from build123d import *

# Parameters (mm, degrees)
F0_R          = 13.5
F0_R_2        = 11.95
F1_DEPTH      = 3.6
F1_DEPTH_BACK = 3.992162
F2_R          = 12.1
F2_R_2        = 11.95
F3_DEPTH      = 2.4
F4_R          = 12.1
F5_DEPTH      = 2.4


with BuildPart() as f1:
    # F0 (on Front) → F1 (new body, two sides)
    with BuildSketch(Plane.XZ) as f1_sk:
        Circle(F0_R)
        Circle(F0_R_2, mode=Mode.SUBTRACT)
    extrude(amount=F1_DEPTH)
    extrude(f1_sk.sketch, amount=-F1_DEPTH_BACK)

    # F2 (on face) → F3 (cut)
    with BuildSketch(Plane.XZ.offset(3.6)):
        Circle(F2_R)
        Circle(F2_R_2, mode=Mode.SUBTRACT)
    extrude(amount=-F3_DEPTH, mode=Mode.SUBTRACT)

    # F4 (on face) → F5 (cut)
    with BuildSketch(Plane(origin=(0, 3.992162, 0), x_dir=(-1, 0, 0), z_dir=(0, 1, 0))):
        Circle(F4_R)
    extrude(amount=-F5_DEPTH, mode=Mode.SUBTRACT)


solid = f1.part
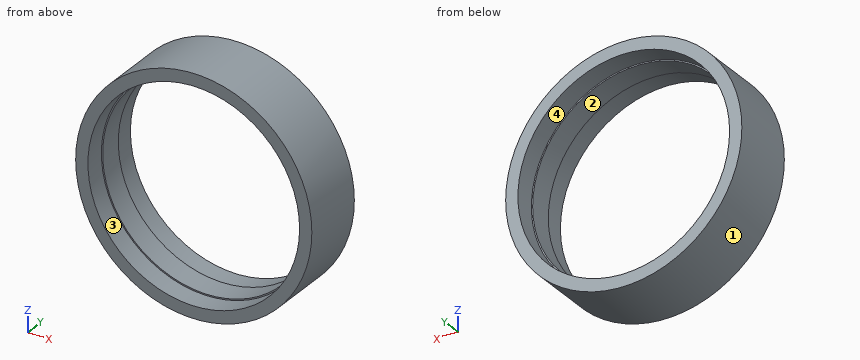
For this review, take the finished solid that the model builds, in its own axes (mm). Face numbers are marked on the shaded views. A direction names the side the tool comes from. Round coordinates to 2 decimals unless told otherwise and drop trailing zeros. Loops run counter-clockwise (first coordinate to the right, second up) from the corner with the lowest first, then second, coordinate; pieces in that order, holes last. Notation, with made-up numbers: (16, 67) - (44, 67) arc R18 ccw to (44, 97) - close; hole circle Ø6 at (3.5, -4.5). An arc over 180 degrees is marked (long way). One line per item, written item: value. Start each with the question number.
Item 1: The part is to be moulded in two halves that separate along X. For the marked faces 1 and 2, say which applies: +X half, -X half, draft (parallel to the pull), parting line (faces both ways), or undercut.
Item 2: For L1, parallel to Z at x = 0, y = 2.1; L2, parallel to Z at x = -9.75, y = -2.5; L3, parallel to X at y = 1.75, z = -1, list the stretches that pass through material, from the lowest coordinate up.
Item 3: Take a section at A-A (z = 0). Give the boundary of the cut face in (x, y).
Item 4: For the marked faces 3 and 4, list the 3-axis set-ups (+Z, -Z, +X, -X, +Y, -Y) from which the entire face can be reached by the end or side of a thin tool; tool diameter is ignored.
Item 5: Take a section at B-B (x = -1). Give the boundary of the cut face in (y, z), plus the area to 3 significant figures.
Item 6: Take a section at C-C (y = 3.25). Give the boundary of the cut face in (x, z).
Item 7: Clearance check with flat-ended pins moving along their axes: pin 1 Ø1.5 at (x, z) = (0, -11) entering from -Y; pin 2 Ø1 at (y, z) = (1.5, -9) entering from +X; pin 3 Ø1.5 at (x, y) = (7, -2) entering from +Z. State where each tip first meets the part, or that it passes through.
Item 8: Take a section at D-D (y = 0.5). Give the boundary of the cut face in (x, z).
Answer below:
1. face 1: parting line
1. face 2: undercut
2. L1: z = -13.5 to -12.1, 12.1 to 13.5
2. L2: z = -9.34 to -7.17, 7.17 to 9.34
2. L3: x = -13.46 to -12.06, 12.06 to 13.46
3. outline: (-13.5, -3.6) - (-12.1, -3.6) - (-12.1, -1.2) - (-11.95, -1.2) - (-11.95, 1.59) - (-12.1, 1.59) - (-12.1, 3.99) - (-13.5, 3.99) - close; (11.95, -1.2) - (12.1, -1.2) - (12.1, -3.6) - (13.5, -3.6) - (13.5, 3.99) - (12.1, 3.99) - (12.1, 1.59) - (11.95, 1.59) - close
4. face 3: -Y
4. face 4: +Y
5. outline: (-3.6, -13.46) - (3.99, -13.46) - (3.99, -12.06) - (1.59, -12.06) - (1.59, -11.91) - (-1.2, -11.91) - (-1.2, -12.06) - (-3.6, -12.06) - close; (-3.6, 12.06) - (-1.2, 12.06) - (-1.2, 11.91) - (1.59, 11.91) - (1.59, 12.06) - (3.99, 12.06) - (3.99, 13.46) - (-3.6, 13.46) - close
5. area: 22.2 mm2
6. outline: circle Ø27 at (0, 0); hole circle Ø24.2 at (0, 0)
7. pin 1: passes through
7. pin 2: stops at x = 10.49
7. pin 3: stops at z = 11.97
8. outline: circle Ø27 at (0, 0); hole circle Ø23.9 at (0, 0)
